Geometry check sheet. Reference: the model listing, model coordinates, mm. A direction names the side the tool comes from. Give positions to 0.01 mm unless a question says otherwise; leave off trailing zeros. Loops run counter-clockwise (first coordinate to the right, second up) from the corner with the lowest first, then second, coordinate; pieces in that order, holes last. Notation, with made-up numbers: (45, 42.5) - (81, 42.5) arc R14 cw to (81, 60.5) - close; hole circle Ø11 at (5, 31). An arc over 180 degrees is marked (long way). Use a Markdown table: item, result. Add a question column.
1. Cross-section at D-D on z = 21. Enter the section's corners in (x, y), and give its area (3 significant figures).
2. Cross-section at B-B on y = -6. Enter the section's corners in (x, z), and give its area (3 significant figures).
3. Set-up check for faces 1 (the flat face through (-23, 12.044, -13)), 2 (the flat face through (-21, -21, -8)), 3 (the flat face through (21, 21, -8)): record each of +Z, -Z, +X, -X, +Y, -Y from which the full face is reachable in a straight line by a thin tool's end or side.
4. Cross-section at A-A on x = 0. Enter the section's corners in (y, z).
5. Draft check along Y on faces 4 (the cylindrical face through (22.11, 11.47, -8.6)), 5 (the cylindrical face through (-0.436, -27.747, -12.563)), 6 (the flat face through (0, -26, -8)), 7 (the conical face through (0.36, -23, -13.25)). Enter one of: pulls with the +Y half, pulls with the -Y half, needs draft (parallel to the pull), parting line crosses it, or undercut.
6. Cross-section at C-C on z = 28. Enter the section's corners in (x, y).
7. Material ranges on L1, parallel to Z at x = -20, y = -23; L2, parallel to Y at x = 0, z = 18.5; L3, parallel to Y at x = 10, z = 26.5, recorded low to high.
8. Depth check by flat-ended pin: P1, Ø2, axis at x = 20, z = -4, coming from the +Y side; P2, Ø1.5, axis at y = 11.5, z = 27.5, coming from the -X side; P3, Ø5, axis at x = -23.5, y = -1, coming from the -Z side; P4, Ø6.5, axis at x = 17, y = -16.5, coming from the -Z side. Enter the tip coordinate at first touch or a pass-through.
from build123d import *
from build123d.topology import SkipClean

# Parameters (mm, degrees)
SKETCH_1_R                  = 24.250000000000004
SKETCH_1_R_2                = 22.75
EXTRUDE_1_DEPTH             = 35
EXTRUDE_START               = 8
SKETCH_2_R                  = 22.75
EXTRUDE_2_DEPTH             = 8
HOLE_WIZARD_M3_1_AT_2_COUNT = 2
HOLE_WIZARD_M3_1_AT_2_PITCH = 40
EXTRUDE_START_2             = 9
EXTRUDE_3_DEPTH             = 9
CUT_EXTRUDE_1_DEPTH         = 52.18654608390758
CUT_EXTRUDE_1_DEPTH_BACK    = 52.18654608390758
SKETCH_6_R                  = 3.5
CHAMFER_2_SIZE              = 4
FILLET_1_R                  = 2


with BuildPart() as part:
    # 草图1 → 凸台-拉伸1 (new body)
    with BuildSketch(Plane.XY):
        Circle(SKETCH_1_R)
        Circle(SKETCH_1_R_2, mode=Mode.SUBTRACT)
    extrude(amount=EXTRUDE_1_DEPTH)

    # 草图2 → 凸台-拉伸2 (add)
    with SkipClean():  # the faces are left unmerged after this step: merging them gives an invalid solid
        with BuildSketch(Plane(origin=(0, 0, 0), x_dir=(-1, 0, 0), z_dir=(0, 0, -1)).offset(EXTRUDE_START)):
            Polygon((-24.999999999999883, -24.999999999999883), (24.999999999999876, -24.999999999999883), (24.999999999999883, 24.999999999999876), (-24.999999999999883, 24.999999999999876), align=None)
            Circle(SKETCH_2_R, mode=Mode.SUBTRACT)
        extrude(amount=-EXTRUDE_2_DEPTH)

    # 草图4 → M3 螺纹孔1 (revolve, cut)
    with SkipClean():  # the faces are left unmerged after this step: merging them gives an invalid solid
        with BuildSketch(Plane(origin=(-20, 24.999999999999876, -4), x_dir=(0, 0, 1), z_dir=(1, 0, 0))):
            Polygon((0, 0), (-1.9e-15, 7.75107577378445), (1.249999999999998, 6.999999999999999), (1.249999999999989, -1.4e-15), align=None)
        hole_wizard_m3_1 = revolve(axis=Axis((-20, 31.349999999999866, -4), (0, -1, 0)), mode=Mode.SUBTRACT)

    # M3 螺纹孔1 at 2: M3 螺纹孔1 ×2
    with SkipClean():  # the faces are left unmerged after this step: merging them gives an invalid solid
        with Locations(*[(i * HOLE_WIZARD_M3_1_AT_2_PITCH, 0, 0) for i in range(1, HOLE_WIZARD_M3_1_AT_2_COUNT)]):
            add(hole_wizard_m3_1, mode=Mode.SUBTRACT)

    # 草图5 → 凸台-拉伸3 (add)
    with SkipClean():  # the faces are left unmerged after this step: merging them gives an invalid solid
        with BuildSketch(Plane(origin=(0, 0, -8), x_dir=(-1, 0, 0), z_dir=(0, 0, -1)).offset(EXTRUDE_START_2)):
            with BuildLine():
                Line((-24.999999999999883, -12.044189470446147), (-19.30025906561863, -12.044189470446147))
                ThreePointArc((-19.30025906561863, -12.044189470446147), (1.39e-15, -22.75), (19.30025906561863, -12.044189470446147))
                Line((19.30025906561863, -12.044189470446147), (24.999999999999883, -12.044189470446147))
                ThreePointArc((24.999999999999883, -12.044189470446147), (1.7e-15, -27.75), (-24.999999999999883, -12.044189470446147))
            make_face()
            with BuildLine():
                Line((24.999999999999883, 12.044189470446147), (19.300259065618633, 12.044189470446147))
                ThreePointArc((19.300259065618633, 12.044189470446147), (6.44e-15, 22.749999999999975), (-19.3002590656186, 12.044189470446147))
                Line((-19.3002590656186, 12.044189470446147), (-24.999999999999854, 12.044189470446147))
                ThreePointArc((-24.999999999999854, 12.044189470446147), (7.86e-15, 27.749999999999975), (24.999999999999883, 12.044189470446147))
            make_face()
        extrude(amount=-EXTRUDE_3_DEPTH)

    # 草图6 → 切除-拉伸1 (cut, two sides: drawn at the far end of the back side and taken through both)
    with SkipClean():  # the faces are left unmerged after this step: merging them gives an invalid solid
        with BuildSketch(Plane(origin=(0, 0, 0), x_dir=(0, 0, -1), z_dir=(1, 0, 0)).offset(-CUT_EXTRUDE_1_DEPTH_BACK)):
            with Locations((-20.999999999999996, 0)):
                Circle(SKETCH_6_R)
        extrude(amount=CUT_EXTRUDE_1_DEPTH + CUT_EXTRUDE_1_DEPTH_BACK, mode=Mode.SUBTRACT)

    # 倒角2
    chamfer_2_edges = [part.edges().sort_by_distance(p)[0] for p in [
        (0, -22.75, -17),
        (-1.599e-14, 22.74999999999998, -17),
    ]]
    chamfer(chamfer_2_edges, length=CHAMFER_2_SIZE)

    # 圆角1
    # the kernel refuses this fillet: 2 mm, written as the material it adds along each edge
    with BuildSketch(Plane(origin=(-14.30025906561863, -12.044189470446147, -8), x_dir=(0, 1, 0), z_dir=(-1, 0, 0))) as fillet_1_piece_1_section:
        with BuildLine():
            CenterArc((FILLET_1_R, FILLET_1_R), FILLET_1_R, 180, 90)
            Line((0, FILLET_1_R), (0, 0))
            Line((0, 0), (FILLET_1_R, 0))
        make_face()
    fillet_1_piece_1 = extrude(amount=10.699740934381254, mode=Mode.PRIVATE)
    fillet_1_piece_1 = fillet_1_piece_1 - Plane(origin=(0, 0, -8.464512968517406), x_dir=(-1, 0, 0), z_dir=(0, 0, -1)) * Cylinder(22.75, 30, mode=Mode.PRIVATE)
    fillet_1_piece_1 = fillet_1_piece_1 & Plane(origin=(0, 0, -8.464512968517406), x_dir=(-0.9009009009008967, -0.43402484578184314, 0), z_dir=(0, 0, -1)) * Cylinder(27.75, 30, mode=Mode.PRIVATE)
    add(fillet_1_piece_1)
    with BuildSketch(Plane(origin=(24.999999999999883, -12.044189470446147, -8), x_dir=(0, 1, 0), z_dir=(-1, 0, 0))) as fillet_1_piece_2_section:
        with BuildLine():
            CenterArc((FILLET_1_R, FILLET_1_R), FILLET_1_R, 180, 90)
            Line((0, FILLET_1_R), (0, 0))
            Line((0, 0), (FILLET_1_R, 0))
        make_face()
    fillet_1_piece_2 = extrude(amount=10.699740934381254, mode=Mode.PRIVATE)
    fillet_1_piece_2 = fillet_1_piece_2 - Plane(origin=(0, 0, -8.464511682363383), x_dir=(-1, 0, 0), z_dir=(0, 0, -1)) * Cylinder(22.75, 30, mode=Mode.PRIVATE)
    fillet_1_piece_2 = fillet_1_piece_2 & Plane(origin=(0, 0, -8.464511682363383), x_dir=(-0.9009009009008967, -0.43402484578184314, 0), z_dir=(0, 0, -1)) * Cylinder(27.75, 30, mode=Mode.PRIVATE)
    add(fillet_1_piece_2)
    with BuildSketch(Plane(origin=(14.3002590656186, 12.044189470446147, -8), x_dir=(0, 0, -1), z_dir=(1, 0, 0))) as fillet_1_piece_3_section:
        with BuildLine():
            CenterArc((FILLET_1_R, -FILLET_1_R), FILLET_1_R, 90, 90)
            Line((0, -FILLET_1_R), (0, 0))
            Line((0, 0), (FILLET_1_R, 0))
        make_face()
    fillet_1_piece_3 = extrude(amount=10.699740934381254, mode=Mode.PRIVATE)
    fillet_1_piece_3 = fillet_1_piece_3 - Plane(origin=(-1.599e-14, -3.197e-14, -8.464512428813396), x_dir=(-0.8483630358513676, 0.5294149217778539, 0), z_dir=(0, 0, -1)) * Cylinder(22.75000000000001, 30, mode=Mode.PRIVATE)
    fillet_1_piece_3 = fillet_1_piece_3 & Plane(origin=(-1.421e-14, -2.487e-14, -8.464512428813396), x_dir=(0.9009009009008963, 0.4340248457818441, 0), z_dir=(0, 0, -1)) * Cylinder(27.75, 30, mode=Mode.PRIVATE)
    add(fillet_1_piece_3)
    with BuildSketch(Plane(origin=(-24.999999999999883, 12.044189470446147, -8), x_dir=(0, 0, -1), z_dir=(1, 0, 0))) as fillet_1_piece_4_section:
        with BuildLine():
            CenterArc((FILLET_1_R, -FILLET_1_R), FILLET_1_R, 90, 90)
            Line((0, -FILLET_1_R), (0, 0))
            Line((0, 0), (FILLET_1_R, 0))
        make_face()
    fillet_1_piece_4 = extrude(amount=10.69974093438125, mode=Mode.PRIVATE)
    fillet_1_piece_4 = fillet_1_piece_4 - Plane(origin=(-1.599e-14, -3.197e-14, -8.464512598097409), x_dir=(-0.8483630358513676, 0.5294149217778539, 0), z_dir=(0, 0, -1)) * Cylinder(22.75000000000001, 30, mode=Mode.PRIVATE)
    fillet_1_piece_4 = fillet_1_piece_4 & Plane(origin=(-1.421e-14, -2.487e-14, -8.464512598097409), x_dir=(0.9009009009008963, 0.4340248457818441, 0), z_dir=(0, 0, -1)) * Cylinder(27.75, 30, mode=Mode.PRIVATE)
    add(fillet_1_piece_4)

    # 镜向1: M3 螺纹孔1 across plane
    add(hole_wizard_m3_1.mirror(Plane.ZX), mode=Mode.SUBTRACT)

    # 镜向1 copy 1 sketch → 镜向1 copy 1 (revolve, cut)
    with BuildSketch(Plane(origin=(20, -24.999999999999876, -4), x_dir=(0, 0, 1), z_dir=(1, 0, 0))):
        Polygon((0, 0), (-1.9e-15, -7.75107577378445), (1.249999999999998, -6.999999999999999), (1.249999999999989, 1.4e-15), align=None)
    revolve(axis=Axis((20, -31.349999999999866, -4), (0, -1, 0)), mode=Mode.SUBTRACT)


solid = part.part
Values found:
| question | item | result |
|---|---|---|
| 1 | outline | (-24, -3.5) arc R24.25 ccw to (24, -3.5) - (22.48, -3.5) arc R22.75 cw to (-22.48, -3.5) - close; (-24, 3.5) - (-22.48, 3.5) arc R22.75 cw to (22.48, 3.5) - (24, 3.5) arc R24.25 ccw to start |
| 1 | area | 200 mm2 |
| 2 | outline | (-25, -8) - (-21.94, -8) - (-21.94, 35) - (-23.5, 35) - (-23.5, 0) - (-25, 0) - close; (21.94, -8) - (25, -8) - (25, 0) - (23.5, 0) - (23.5, 35) - (21.94, 35) - close |
| 2 | area | 157 mm2 |
| 3 | face 1 | -Z, +X, -X |
| 3 | face 2 | -Z, -X, -Y |
| 3 | face 3 | -Z, +X, +Y |
| 4 | outline | (-27.75, -17) - (-26.75, -17) - (-22.75, -13) - (-22.75, 35) - (-24.25, 35) - (-24.25, 0) - (-25, 0) - (-25, -8) - (-27.75, -8) - close; (22.75, -13) - (26.75, -17) - (27.75, -17) - (27.75, -8) - (25, -8) - (25, 0) - (24.25, 0) - (24.25, 35) - (22.75, 35) - close |
| 5 | face 4 | undercut |
| 5 | face 5 | pulls with the -Y half |
| 5 | face 6 | needs draft |
| 5 | face 7 | undercut |
| 6 | outline | circle Ø48.5 at (0, 0); hole circle Ø45.5 at (0, 0) |
| 7 | L1 | z = -8 to -5.25, -2.75 to 0 |
| 7 | L2 | y = -24.25 to -22.75, 22.75 to 24.25 |
| 7 | L3 | y = -22.09 to -20.43, 20.43 to 22.09 |
| 8 | P1 | stops at y = 17.85 |
| 8 | P2 | stops at x = -21.74 |
| 8 | P3 | stops at z = -8 |
| 8 | P4 | stops at z = -17 |
